```python
from build123d import *

# Parameters (mm, degrees)
SKETCH3_R                       = 2.38125
BOSS_EXTRUDE1_DEPTH             = 55.5625
FILLET2_R                       = 1.5875
F_3_32_0_09375_DIAMETER_HOLE3_D = 2.38125
FILLET3_R                       = 1.5875


with BuildPart() as part:
    # Sketch3 → Boss-Extrude1 (new, symmetric)
    with BuildSketch(Plane.XY):
        Circle(SKETCH3_R)
    extrude(amount=BOSS_EXTRUDE1_DEPTH, both=True)

    # Fillet2
    fillet2_edges = [part.edges().sort_by_distance(p)[0] for p in [
        (-2.38125, 0, 55.5625),
    ]]
    fillet(fillet2_edges, radius=FILLET2_R)

    # 3/32 (0.09375) Diameter Hole3 (through all)
    with Locations(Plane(origin=(0, 2.38125, 0), x_dir=(1, 0, 0), z_dir=(0, 1, 0))):
        with Locations((0, 52.3875)):
            Hole(F_3_32_0_09375_DIAMETER_HOLE3_D / 2)

    # Fillet3
    fillet3_edges = [part.edges().sort_by_distance(p)[0] for p in [
        (-2.38125, 0, -55.5625),
    ]]
    fillet(fillet3_edges, radius=FILLET3_R)


solid = part.part
```
Verification items for the finished model (mm, model axes). Round coordinates to 2 decimals unless told otherwise and drop trailing zeros. Order: outer loops, then holes, each group sorted by start corner. A loop starts at its lowest first (then second) coordinate and runs counter-clockwise, first axis right, second up.
1) Depth check by flat-ended pin: pin 1 (1 mm diameter, centred on y = -2, z = -13.5, fed in from -X). Enter the tip coordinate at first touch or a pass-through.
Geometry says:
pin 1: stops at x = -1.85
2) Material ranges on line 1 (Z direction, x = 0, y = -0.35); line 2 (X direction, y = -0.25, z = 18); line 3 (Z direction, x = 0, y = 1), recorded low to high.
Geometry says:
line 1: z = -55.56 to -53.58, -51.2 to 55.56
line 2: x = -2.37 to 2.37
line 3: z = -55.55 to -53.58, -51.2 to 55.55
3) Cross-section at A-A, the plane z = -41.5. Record the cut outline in (x, y), plus the area to 3 significant figures.
Geometry says:
outline: circle Ø4.76 at (0, 0)
area: 17.8 mm2
